Source: CAD feature listing. Evaluate the final solid. Frame: model axes, mm. A direction names the side the tool comes from. Round coordinates to 2 decimals unless told otherwise and drop trailing zeros. Loops run counter-clockwise (first coordinate to the right, second up) from the corner with the lowest first, then second, coordinate; pieces in that order, holes last. Notation, with made-up numbers: (36, 18) - (57, 18) arc R24 ccw to (57, 57) - close; hole circle Ø5 at (51, 47.5). An arc over 180 degrees is marked (long way). One line per question, with ' | ' between items. Start each with the question number.
1. Pin query (flat end, axial travel): pin 1 (1 mm diameter, centred on y = 5, z = 0.5, fed in from -X); pin 2 (1.5 mm diameter, centred on x = -0.5, y = -4.5, fed in from +Z) (3 decimals). Return the tip coordinate at first contact, or that it passes through.
2. Cut plane C-C (y = 0.75). Return loops of the section in (x, z) (3 decimals).
3. Ray query, line 1 (Y direction, x = -1.5, z = 1.15); line 2 (Z direction, x = -0.75, y = 3) (3 decimals); line 3 (X direction, y = 6, z = 0.1) (3 decimals). Return the intervals inside material, ascending.
4. Cut plane B-B (z = 0.8). Return loops of the section in (x, y) (3 decimals).
5. Mould query, pull axis X, two halves, no side actions, for faces 5 (the flat face through (-1.975, 6, 0)), 6 (the cylindrical face through (5.474, 0.09, -0.007)), 7 (the cylindrical face through (-3, 0, 0)). Classes: pulls with the +X half, pulls with the -X half, needs draft (parallel to the pull), parting line crosses it, or undercut.
6. Cut plane A-A (x = -0.25). Return loops of the section in (y, z) (3 decimals), then the cut area to 3 significant figures.
7. Cut plane D-D (x = 3.5). Return loops of the section in (y, z) (3 decimals).
8. Access query for faces 1 (the flat face through (0, -6.3, 1)), 2 (the flat face through (1.975, -6, 0)), 3 (the flat face through (0, 6, 0.375)), 4 (the flat face through (0, 2.5, 0)). Directions: +Z, -Z, +X, -X, +Y, -Y. A direction counts if a zero-diameter tool reaches every point of the face in a straight line with its end or side. Return the directions, or none.
Autodesk Inventor part; units mm, degrees
ref_plane "YZ Plane" through (0, 0, 0) normal (1, 0, 0) x (0, 1, 0)
ref_plane "XZ Plane" through (0, 0, 0) normal (0, 1, 0) x (-1, 0, 0)
ref_plane "XY Plane" through (0, 0, 0) normal (0, 0, 1) x (1, 0, 0)
sketch "Szkic4" plane through (0, 0, 0) normal (0, 0, 1) x (1, 0, 0)
  line L0 (-1.6583, 2.5) -> (1.6583, 2.5)
  line L1 (-1.6583, -2.5) -> (1.6583, -2.5)
  arc A0 (-1.6583, 2.5) -> (-1.6583, -2.5) centre (0, 0) ccw
  arc A1 (1.6583, -2.5) -> (1.6583, 2.5) centre (0, 0) ccw
  line L2 (-1.975, 7.25) -> (1.975, 7.25)
  line L3 (-1.975, 7.25) -> (-1.975, 5.2749)
  line L4 (1.975, 7.25) -> (1.975, 5.2749)
  arc A2 (1.975, 5.2749) -> (2.1278, 5.0446) centre (2.225, 5.2749) ccw
  arc A3 (-2.1278, 5.0446) -> (-1.975, 5.2749) centre (-2.225, 5.2749) ccw
  line L5 (-1.975, -7.25) -> (1.975, -7.25)
  line L6 (-1.975, -7.25) -> (-1.975, -5.2749)
  line L7 (1.975, -7.25) -> (1.975, -5.2749)
  arc A4 (2.1278, -5.0446) -> (1.975, -5.2749) centre (2.225, -5.2749) ccw
  arc A5 (-1.975, -5.2749) -> (-2.1278, -5.0446) centre (-2.225, -5.2749) ccw
  arc A6 (-2.1278, 5.0446) -> (-2.1278, -5.0446) centre (0, 0) ccw
  arc A7 (2.1278, -5.0446) -> (2.1278, 5.0446) centre (0, 0) ccw
  point P0 (-1.975, 5.1064)
  point P1 (1.975, 5.1064)
  point P2 (-1.975, -5.1064)
  point P3 (1.975, -5.1064)
  dimension "d19" = 3.95
  dimension "d20" = 0.25
extrude "Wyciągnięcie proste4" add sketch "Szkic4" along normal mid plane 0.95
sketch "Szkic5" plane through (0, 0, 0.475) normal (0, 0, 1) x (1, 0, 0)
  line L0 (-1.975, 7.25) -> (1.975, 7.25)
  line L1 (1.975, 7.25) -> (1.975, 6.404)
  line L2 (1.975, 6.404) -> (-1.975, 6.404)
  line L3 (-1.975, 6.404) -> (-1.975, 7.25)
  line L4 (1.975, -7.25) -> (-1.975, -7.25)
  line L5 (-1.975, -7.25) -> (-1.975, -6.3)
  line L6 (-1.975, -6.3) -> (1.975, -6.3)
  line L7 (1.975, -6.3) -> (1.975, -7.25)
  dimension "d23" = 0.95
extrude "Wyciągnięcie proste5" add sketch "Szkic5" along normal blind 1.35
fillet "Zaokrąglenie3" radius 0.95 2 edges at (0, 7.25, -0.475) (0, -7.25, -0.475)
sketch "Szkic6" plane through (0, 0, 0.475) normal (0, 0, 1) x (1, 0, 0)
  line L0 (-1.475, 5.2749) -> (1.475, 5.2749)
  line L1 (1.475, 5.2749) -> (1.475, 6.404)
  line L2 (1.475, 6.404) -> (-1.475, 6.404)
  line L3 (-1.475, 6.404) -> (-1.475, 5.2749)
  line L4 (-1.475, -5.2749) -> (1.475, -5.2749)
  line L5 (1.475, -5.2749) -> (1.475, -6.404)
  line L6 (1.475, -6.404) -> (-1.475, -6.404)
  line L7 (-1.475, -6.404) -> (-1.475, -5.2749)
extrude "Wyciągnięcie proste6" cut sketch "Szkic6" against normal blind 0.1
properties part number "podkładka z dwoma uszami" material "Stal"
Answers follow:
1) pin 1: stops at x = -3.12 | pin 2: stops at z = 0.475
2) outline: (-5.423, -0.475) - (-2.905, -0.475) - (-2.905, 0.475) - (-5.423, 0.475) - close; (2.905, -0.475) - (5.423, -0.475) - (5.423, 0.475) - (2.905, 0.475) - close
3) line 1: y = -7.25 to -6.3, 6.4 to 7.25 | line 2: z = -0.475 to 0.475 | line 3: x = -1.975 to 1.975
4) outline: (-1.975, -7.25) - (1.975, -7.25) - (1.975, -6.3) - (-1.975, -6.3) - close; (-1.975, 6.404) - (1.975, 6.404) - (1.975, 7.25) - (-1.975, 7.25) - close
5) face 5: pulls with the -X half | face 6: pulls with the +X half | face 7: undercut
6) outline: (-7.25, 0.475) arc R0.95 ccw to (-6.3, -0.475) - (-2.5, -0.475) - (-2.5, 0.475) - (-5.275, 0.475) - (-5.275, 0.375) - (-6.404, 0.375) - (-6.404, 0.475) - (-6.3, 0.475) - (-6.3, 1.825) - (-7.25, 1.825) - close; (2.5, -0.475) - (6.3, -0.475) arc R0.95 ccw to (7.25, 0.475) - (7.25, 1.825) - (6.404, 1.825) - (6.404, 0.375) - (5.275, 0.375) - (5.275, 0.475) - (2.5, 0.475) - close | area: 10.8 mm2
7) outline: (-4.21, -0.475) - (4.21, -0.475) - (4.21, 0.475) - (-4.21, 0.475) - close
8) face 1: +Z, +X, -X | face 2: +Z, -Z, +X, -Y | face 3: +Z | face 4: +Z, -Z
